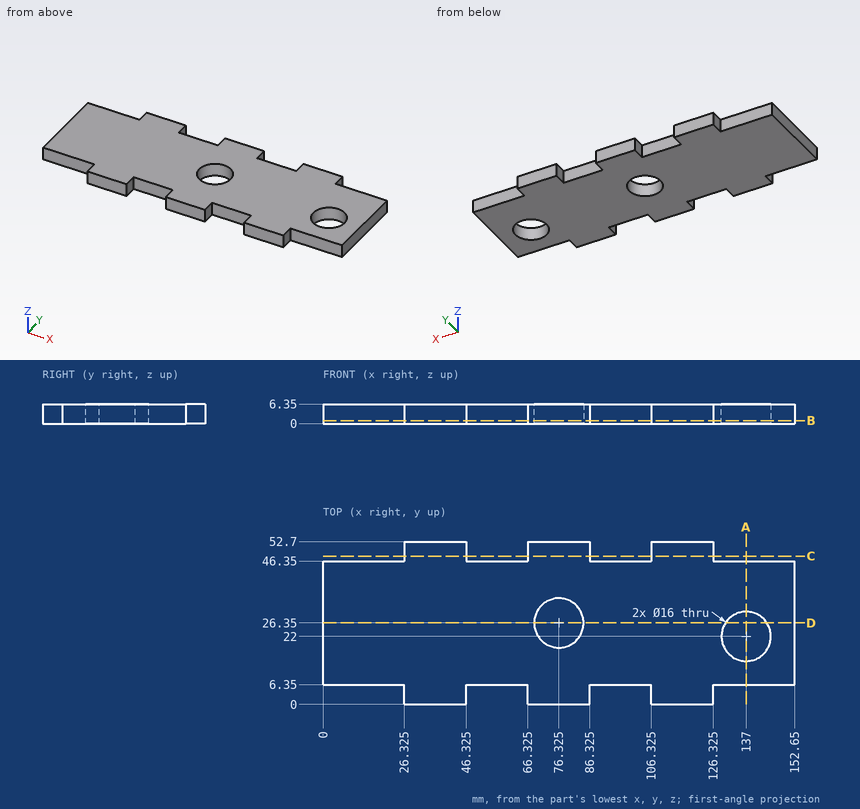
The figure shows three views and two pictorial views of one solid part (mm, origin at its lowest corner). Answer the questions. Give positions to 0.01 mm unless a question says otherwise; leave off trailing zeros. Loops run counter-clockwise (first coordinate to the right, second up) from the corner with the lowest first, then second, coordinate; pieces in that order, holes last. Notation, with made-up numbers: (-0.75, 39.25) -> (15.25, 39.25) arc R22 cw to (15.25, 75.25) -> close; hole circle Ø8 at (39.5, 7.25). An arc over 180 degrees is marked (long way). Put each result on its own line as item: value. Start each with the question number.
Item 1: The part is cut by section D-D (y = 26.35). Give the vertices of the cut face in (x, z) (3 decimals), then the cut area to 3 significant figures.
Item 2: The part is cut by section B-B (z = 1). State how many separate pieces and enclosed holes the cut face has, then the cut area to 3 significant figures.
Item 3: Each of these flat-tipped pins is pushed along its axis until it touches: P1, Ø3, axis at y = 3, z = 2.5, coming from the +X side (3 decimals); P2, Ø1.9, axis at x = 93.5, z = 4, coming from the -Y side; P3, Ø3, axis at x = 98, z = 2.5, coming from the +Y side; P4, Ø1, axis at x = 101, y = 38.5, coming from the -Z side. Where does it stop, or does it pass through?
Item 4: The part is cut by section C-C (y = 48). Give the vertices of the cut face in (x, z) (3 decimals).
Item 5: Find the intervals of material crossed by L1, parallel to X at y = 49, z = 3 (3 decimals); L2, parallel to Y at x = 137, z = 2; L3, parallel to X at y = 19, z = 0.5, in increasing order. Write a range as [from, to].
Item 6: The part is cut by section A-A (x = 137). Give the vertices of the cut face in (y, z).
Answers below:
1. outline: (0, 0) -> (68.325, 0) -> (68.325, 6.35) -> (0, 6.35) -> close; (84.325, 0) -> (130.286, 0) -> (130.286, 6.35) -> (84.325, 6.35) -> close; (143.714, 0) -> (152.65, 0) -> (152.65, 6.35) -> (143.714, 6.35) -> close
1. area: 782 mm2
2. separate pieces: 1
2. enclosed holes: 2
2. area: 6,470 mm2
3. P1: x = 126.325
3. P2: y = 6.35
3. P3: y = 46.35
3. P4: z = 0
4. outline: (26.325, 0) -> (46.325, 0) -> (46.325, 6.35) -> (26.325, 6.35) -> close; (66.325, 0) -> (86.325, 0) -> (86.325, 6.35) -> (66.325, 6.35) -> close; (106.325, 0) -> (126.325, 0) -> (126.325, 6.35) -> (106.325, 6.35) -> close
5. L1: [26.325, 46.325], [66.325, 86.325], [106.325, 126.325]
5. L2: [6.35, 14], [30, 46.35]
5. L3: [0, 73.17], [79.48, 129.58], [144.42, 152.65]
6. outline: (6.35, 0) -> (14, 0) -> (14, 6.35) -> (6.35, 6.35) -> close; (30, 0) -> (46.35, 0) -> (46.35, 6.35) -> (30, 6.35) -> close
